```python
from build123d import *

# Parameters (mm, degrees)
F0_W     = 50
F0_H     = 10
F1_DEPTH = 1
F3_DEPTH = 25
F4_R     = 1


with BuildPart() as f1:
    # F0 (on Top) → F1 (new body)
    with BuildSketch(Plane.XY):
        with Locations((25, 5)):
            Rectangle(F0_W, F0_H)
    extrude(amount=F1_DEPTH)

    # F2 (on face) → F3 (cut)
    with BuildSketch(Plane.XY.offset(1)):
        with BuildLine():
            Line((21, 6.65), (4, 6.65))
            ThreePointArc((4, 6.65), (2.35, 5), (4, 3.35))
            Line((4, 3.35), (21, 3.35))
            ThreePointArc((21, 3.35), (22.65, 5), (21, 6.65))
        make_face()
        with BuildLine():
            ThreePointArc((29, 6.65), (27.35, 5), (29, 3.35))
            Line((29, 3.35), (46, 3.35))
            ThreePointArc((46, 3.35), (47.65, 5), (46, 6.65))
            Line((46, 6.65), (29, 6.65))
        make_face()
    extrude(amount=-F3_DEPTH, mode=Mode.SUBTRACT)

    # F4
    f4_edges = [f1.edges().sort_by_distance(p)[0] for p in [
        (50, 0, 0.5),
        (50, 10, 0.5),
        (0, 10, 0.5),
        (0, 0, 0.5),
    ]]
    fillet(f4_edges, radius=F4_R)


solid = f1.part
```
The listing builds one solid part. Answer for the finished solid, in the listing's coordinates (mm). A direction names the side the tool comes from. Round coordinates to 2 decimals unless told otherwise and drop trailing zeros. Loops run counter-clockwise (first coordinate to the right, second up) from the corner with the lowest first, then second, coordinate; pieces in that order, holes last.
Q1. Section D-D, the plane x = 47 is taken. Determine the outline of the cut face in (y, z), then the cut area to 3 significant figures.
Q2. Section A-A, the plane y = 5 is taken. Determine the outline of the cut face in (x, z), then the cut area to 3 significant figures.
Q3. Section B-B, the plane x = 38.5 is taken. Determine the outline of the cut face in (y, z).
Q4. Which of the six approach directions +Z, -Z, +X, -X, +Y, -Y give full straight-line access (tool end or side, diameter ignored) to faces 1 (the face through (37.4, 3.35, 0.5)), 2 (the face through (49.699, 0.285, 0.507))?
Q5. For a pull along X with two mould halves and no side action, classify faces 3 (the face through (47.65, 4.96, 0.51)), 4 (the face through (0, 4.9, 0.5)), 5 (the face through (24.7, 0, 0.5)), 6 (the face through (37.6, 6.65, 0.5)) as released by +X, released by -X, zero draft, split by the parting line, or undercut.
Q6. Section C-C, the plane z = 0.4 is taken. Determine the outline of the cut face in (x, y).
Q7. Find the intervals of material crossed by line 1 (X direction, y = 5, z = 0.9); line 2 (Y direction, x = 15, z = 0.65); line 3 (X direction, y = 6.5, z = 0.9), in increasing order.
Completed:
1. outline: (0, 0) - (3.69, 0) - (3.69, 1) - (0, 1) - close; (6.31, 0) - (10, 0) - (10, 1) - (6.31, 1) - close
1. area: 7.38 mm2
2. outline: (0, 0) - (2.35, 0) - (2.35, 1) - (0, 1) - close; (22.65, 0) - (27.35, 0) - (27.35, 1) - (22.65, 1) - close; (47.65, 0) - (50, 0) - (50, 1) - (47.65, 1) - close
2. area: 9.40 mm2
3. outline: (0, 0) - (3.35, 0) - (3.35, 1) - (0, 1) - close; (6.65, 0) - (10, 0) - (10, 1) - (6.65, 1) - close
4. face 1: +Z, -Z
4. face 2: +Z, -Z, +X, -Y
5. face 3: undercut
5. face 4: released by -X
5. face 5: zero draft
5. face 6: undercut
6. outline: (0, 1) arc R1 ccw to (1, 0) - (49, 0) arc R1 ccw to (50, 1) - (50, 9) arc R1 ccw to (49, 10) - (1, 10) arc R1 ccw to (0, 9) - close; hole (4, 3.35) - (21, 3.35) arc R1.65 ccw to (21, 6.65) - (4, 6.65) arc R1.65 ccw to start; hole (29, 3.35) - (46, 3.35) arc R1.65 ccw to (46, 6.65) - (29, 6.65) arc R1.65 ccw to start
7. line 1: x = 0 to 2.35, 22.65 to 27.35, 47.65 to 50
7. line 2: y = 0 to 3.35, 6.65 to 10
7. line 3: x = 0 to 3.31, 21.69 to 28.31, 46.69 to 50
